from build123d import *

# Parameters (mm, degrees)
MODEL_R             = 1.500000002
BOSS_EXTRUDE1_DEPTH = 3


with BuildPart() as part:
    # Model → Boss-Extrude1 (new body)
    with BuildSketch(Plane.XY):
        with BuildLine():
            Line((67.745687083, 17.48726701), (67.745687083, 21.23726701))
            Line((67.745687083, 21.23726701), (71.745687083, 21.23726701))
            Line((71.745687083, 21.23726701), (71.745687083, 19.98726701))
            Line((71.745687083, 19.98726701), (74.245687083, 19.98726701))
            Line((74.245687083, 19.98726701), (74.245687083, 21.23726701))
            Line((74.245687083, 21.23726701), (77.745687083, 21.23726701))
            Line((77.745687083, 21.23726701), (77.745687083, 24.23726701))
            Line((77.745687083, 24.23726701), (74.245687083, 24.23726701))
            Line((74.245687083, 24.23726701), (74.245687083, 25.48726701))
            Line((74.245687083, 25.48726701), (71.745687083, 25.48726701))
            Line((71.745687083, 25.48726701), (71.745687083, 24.23726701))
            Line((71.745687083, 24.23726701), (67.745687083, 24.23726701))
            Line((67.745687083, 24.23726701), (67.924311205, 28.98726701))
            Line((67.924311205, 28.98726701), (68.995687083, 28.98726701))
            Line((68.995687083, 28.98726701), (84.745617476, 28.98726701))
            Line((84.745617476, 28.98726701), (84.745617476, 65.48726701))
            Line((84.745617476, 65.48726701), (89.245617476, 65.48726701))
            Line((89.245617476, 65.48726701), (89.245617476, 68.48726701))
            Line((89.245617476, 68.48726701), (99.376117267, 68.48726701))
            Line((99.376117267, 68.48726701), (99.376117267, 65.487488154))
            Line((99.376117267, 65.487488154), (99.376117267, 30.302957894))
            ThreePointArc((99.376117267, 30.302957894), (100.4489582, 24.623653509), (96.229587083, 20.67366701))
            Line((96.229587083, 20.67366701), (83.745687083, 17.48726701))
            Line((83.745687083, 17.48726701), (79.245687083, 17.48726701))
            Line((79.245687083, 17.48726701), (79.245687083, 14.48726701))
            Line((79.245687083, 14.48726701), (69.245690135, 14.48726701))
            Line((69.245690135, 14.48726701), (69.245687083, 17.48726701))
            Line((69.245687083, 17.48726701), (67.745687083, 17.48726701))
        make_face()
        with Locations((94.745687081, 26.487267012)):
            Circle(MODEL_R, mode=Mode.SUBTRACT)
    extrude(amount=BOSS_EXTRUDE1_DEPTH)


solid = part.part
Work out the finished part from the listing and answer in its coordinate system (mm). A direction names the side the tool comes from. Give positions to 0.01 mm unless a question says otherwise; leave off trailing zeros. Order: outer loops, then holes, each group sorted by start corner. A loop starts at its lowest first (then second) coordinate and runs counter-clockwise, first axis right, second up. Notation, with made-up numbers: (-13.75, -6) -> (-5.75, -6) arc R18 cw to (-5.75, 6) -> close; hole circle Ø2 at (87, 0). An arc over 180 degrees is marked (long way). Answer as a JSON object with one key per item and string values. Group by question number.
1. Section C-C on y = 46 is taken. Determine the outline of the cut face in (x, z), plus the area to 3 significant figures.
2. A tool of negligible diameter and unlimited length cuts with its end or side. For faces 4 (the flat face through (70, 24.237, 1)), 5 (the flat face through (82, 17.487, 1)), 6 (the flat face through (74.246, 21, 1)), 7 (the flat face through (87, 65.487, 1)), from which of +Z, -Z, +X, -X, +Y, -Y can it reach the whole face along a straight path? Write none if from no direction.
3. Section B-B on z = 1.2 is taken. Determine the outline of the cut face in (x, y).
4. Section A-A on x = 76 is taken. Determine the outline of the cut face in (y, z).
5. Flat-ended cylindrical pins translate along their axes: pin 1 Ø0.9 at (y, z) = (66.5, 2) entering from -X; pin 2 Ø0.6 at (y, z) = (24.5, 1.5) entering from +X; pin 3 Ø1 at (y, z) = (44, 0.5) entering from -X. Find the tip coordinate at first contact, or state that the pin passes through.
6. Section D-D on x = 97 is taken. Determine the outline of the cut face in (y, z).
7. The mould has two halves that part along Y. Classify faces 1 (the flat face through (73, 19.987, 1)), 2 (the flat face through (92, 42, 3)), 3 (the flat face through (74, 14.487, 1)): released by +Y, released by -Y, zero draft, split by the parting line, or undercut.
8. Consider line 1 along X through (y, z) = (58, 0.75); line 2 along Y through (x, z) = (93.5, 1.75); line 3 along Y through (x, z) = (78.5, 2.1). Determine where each line is inside the solid, lowest interval first. Write a range as [from, to].
Result sheet:
{
 "1": {"outline": "(84.75, 0) -> (99.38, 0) -> (99.38, 3) -> (84.75, 3) -> close", "area": "43.9 mm^2"},
 "2": {"face 4": "+Z, -Z, -X", "face 5": "+Z, -Z, +X, -Y", "face 6": "+Z, -Z", "face 7": "+Z, -Z, -X, +Y"},
 "3": {"outline": "(67.75, 17.49) -> (69.25, 17.49) -> (69.25, 14.49) -> (79.25, 14.49) -> (79.25, 17.49) -> (83.75, 17.49) -> (96.23, 20.67) arc R6 ccw to (99.38, 30.3) -> (99.38, 68.49) -> (89.25, 68.49) -> (89.25, 65.49) -> (84.75, 65.49) -> (84.75, 28.99) -> (67.92, 28.99) -> (67.75, 24.24) -> (71.75, 24.24) -> (71.75, 25.49) -> (74.25, 25.49) -> (74.25, 24.24) -> (77.75, 24.24) -> (77.75, 21.24) -> (74.25, 21.24) -> (74.25, 19.99) -> (71.75, 19.99) -> (71.75, 21.24) -> (67.75, 21.24) -> close; hole circle Ø3 at (94.75, 26.49)"},
 "4": {"outline": "(14.49, 0) -> (21.24, 0) -> (21.24, 3) -> (14.49, 3) -> close; (24.24, 0) -> (28.99, 0) -> (28.99, 3) -> (24.24, 3) -> close"},
 "5": {"pin 1": "stops at x = 89.25", "pin 2": "stops at x = 100.5", "pin 3": "stops at x = 84.75"},
 "6": {"outline": "(20.93, 0) -> (68.49, 0) -> (68.49, 3) -> (20.93, 3) -> close"},
 "7": {"face 1": "undercut", "face 2": "zero draft", "face 3": "released by -Y"},
 "8": {"line 1": "x = [84.75, 99.38]", "line 2": "y = [19.98, 25.65], [27.32, 68.49]", "line 3": "y = [14.49, 28.99]"}
}
